Geometry check sheet. Reference: the model listing, model coordinates, mm. Give positions to 0.01 mm unless a question says otherwise; leave off trailing zeros. Write each loop counter-clockwise with the first axis right and the second up, starting at its lowest first coordinate (ties: lowest second). Pieces come first, ordered by that corner, then holes. Notation, with made-up numbers: (47, 57) -> (53, 57) arc R4 cw to (53, 63) -> close; hole circle Ø4 at (46.25, 62.25). An arc over 180 degrees is marked (long way). One line per item, written item: value.
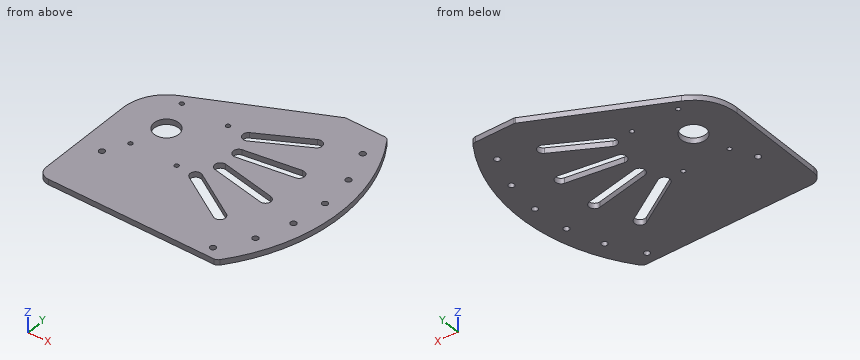
from build123d import *

# Parameters (mm, degrees)
SKETCH1_R           = 3.3782
SKETCH1_R_2         = 14.2875
BOSS_EXTRUDE1_DEPTH = 6.35
FILLET1_R           = 3.175
SKETCH2_R           = 2.54
CUT_EXTRUDE1_DEPTH  = 6.35


with BuildPart() as part:
    # Sketch1 → Boss-Extrude1 (new body)
    with BuildSketch(Plane.XY):
        with BuildLine():
            ThreePointArc((155.542598667, -127), (158.336226208, -126.352468339), (160.56010185, -124.541935484))
            ThreePointArc((160.56010185, -124.541935484), (203.040311847, -8.054301034), (169.920839989, 111.432258065))
            ThreePointArc((169.920839989, 111.432258065), (167.628276357, 113.537255082), (164.61081374, 114.3))
            Line((164.61081374, 114.3), (119.1365603, 114.3))
            Line((119.1365603, 114.3), (-22.183826694, 45.70030452))
            ThreePointArc((-22.183826694, 45.70030452), (-43.055652335, 26.960170659), (-50.8, 0))
            Line((-50.8, 0), (-50.8, -114.3))
            ThreePointArc((-50.8, -114.3), (-47.080256121, -123.280256121), (-38.1, -127))
            Line((-38.1, -127), (155.542598667, -127))
        make_face()
        with Locations((144.383975911, -114.3)):
            Circle(SKETCH1_R, mode=Mode.SUBTRACT)
        with Locations((166.325065928, -79.042592339)):
            Circle(SKETCH1_R, mode=Mode.SUBTRACT)
        with Locations((179.808375328, -39.76541584)):
            Circle(SKETCH1_R, mode=Mode.SUBTRACT)
        with Locations((184.148262492, 1.5342404)):
            Circle(SKETCH1_R, mode=Mode.SUBTRACT)
        with Locations((179.124039222, 42.756241887)):
            Circle(SKETCH1_R, mode=Mode.SUBTRACT)
        with Locations((164.991192987, 81.804402963)):
            Circle(SKETCH1_R, mode=Mode.SUBTRACT)
        with BuildLine():
            Line((63.70579448, 42.288701206), (119.344293443, 72.892743964))
            ThreePointArc((119.344293443, 72.892743964), (127.968547615, 70.389298344), (125.465101994, 61.765044172))
            Line((125.465101994, 61.765044172), (69.826603031, 31.161001414))
            ThreePointArc((69.826603031, 31.161001414), (61.202348859, 33.664447034), (63.70579448, 42.288701206))
        make_face(mode=Mode.SUBTRACT)
        with BuildLine():
            ThreePointArc((61.899520347, -44.891111378), (59.755440765, -36.170565366), (68.475986777, -34.026485785))
            Line((68.475986777, -34.026485785), (122.799114746, -66.908817936))
            ThreePointArc((122.799114746, -66.908817936), (124.943194328, -75.629363948), (116.222648316, -77.77344353))
            Line((116.222648316, -77.77344353), (61.899520347, -44.891111378))
        make_face(mode=Mode.SUBTRACT)
        with BuildLine():
            ThreePointArc((73.520186848, -21.01296328), (68.52280869, -13.551648949), (75.984123021, -8.554270791))
            Line((75.984123021, -8.554270791), (138.277585466, -20.873951654))
            ThreePointArc((138.277585466, -20.873951654), (143.274963624, -28.335265985), (135.813649293, -33.332644143))
            Line((135.813649293, -33.332644143), (73.520186848, -21.01296328))
        make_face(mode=Mode.SUBTRACT)
        with BuildLine():
            ThreePointArc((76.273233773, 5.399658308), (69.025314597, 10.701796332), (74.327452622, 17.949715507))
            Line((74.327452622, 17.949715507), (137.077738619, 27.678621264))
            ThreePointArc((137.077738619, 27.678621264), (144.325657795, 22.37648324), (139.02351977, 15.128564064))
            Line((139.02351977, 15.128564064), (76.273233773, 5.399658308))
        make_face(mode=Mode.SUBTRACT)
        Circle(SKETCH1_R_2, mode=Mode.SUBTRACT)
        with Locations((-25.4, -63.5)):
            Circle(SKETCH1_R, mode=Mode.SUBTRACT)
    extrude(amount=BOSS_EXTRUDE1_DEPTH)

    # Fillet1
    fillet1_edges = [part.edges().sort_by_distance(p)[0] for p in [
        (119.1365603, 114.3, 3.175),
    ]]
    fillet(fillet1_edges, radius=FILLET1_R)

    # Sketch2 → Cut-Extrude1 (cut)
    with BuildSketch(Plane.XY.offset(6.35)):
        with Locations((-12.072682951, 38.1)):
            Circle(SKETCH2_R)
        with Locations((-12.072682951, -38.1)):
            Circle(SKETCH2_R)
        with Locations((41.902317049, -38.1)):
            Circle(SKETCH2_R)
        with Locations((41.902317049, 38.1)):
            Circle(SKETCH2_R)
    extrude(amount=-CUT_EXTRUDE1_DEPTH, mode=Mode.SUBTRACT)


solid = part.part
1) Scan lines: probe 1 along Y at (x, z) = (78, 2.5); probe 2 along Y at (x, z) = (94, 2.5); probe 3 along Y at (x, z) = (137, 4). Record each from-to range of solid material in increasing order.
Verdict:
probe 1: -127 to -54.64, -39.79 to -21.9, -8.95 to 5.67, 18.52 to 35.66, 50.15 to 94.33
probe 2: -127 to -64.32, -49.48 to -25.06, -12.12 to 8.15, 21 to 44.46, 58.95 to 102.1
probe 3: -127 to -33.45, -20.62 to 14.81, 27.67 to 114.3
2) Sectioned sample at C-C on y = -63.5. Record the cut outline in (x, z).
Verdict:
outline: (-50.8, 0) -> (-28.78, 0) -> (-28.78, 6.35) -> (-50.8, 6.35) -> close; (-22.02, 0) -> (92.64, 0) -> (92.64, 6.35) -> (-22.02, 6.35) -> close; (117.17, 0) -> (193.02, 0) -> (193.02, 6.35) -> (117.17, 6.35) -> close
3) Sectioned sample at D-D on x = -25.4. Record the cut outline in (y, z), plus the area to 3 significant figures.
Verdict:
outline: (-127, 0) -> (-66.88, 0) -> (-66.88, 6.35) -> (-127, 6.35) -> close; (-60.12, 0) -> (43.99, 0) -> (43.99, 6.35) -> (-60.12, 6.35) -> close
area: 1,040 mm^2
4) Depth check by flat-ended pin: pin 1 Ø1.5 at (y, z) = (56, 4) entering from -X; pin 2 Ø1.5 at (y, z) = (-50, 3) entering from +X. Enter the tip coordinate at first touch or a pass-through.
Verdict:
pin 1: x = -2.51
pin 2: x = 197.14
5) Sectioned sample at A-A on x = 91.5. Record the cut outline in (y, z).
Verdict:
outline: (-127, 0) -> (-62.81, 0) -> (-62.81, 6.35) -> (-127, 6.35) -> close; (-47.96, 0) -> (-24.57, 0) -> (-24.57, 6.35) -> (-47.96, 6.35) -> close; (-11.62, 0) -> (7.76, 0) -> (7.76, 6.35) -> (-11.62, 6.35) -> close; (20.61, 0) -> (43.08, 0) -> (43.08, 6.35) -> (20.61, 6.35) -> close; (57.58, 0) -> (100.88, 0) -> (100.88, 6.35) -> (57.58, 6.35) -> close
6) Sectioned sample at B-B on x = 5.5. Record the cut outline in (y, z).
Verdict:
outline: (-127, 0) -> (-13.19, 0) -> (-13.19, 6.35) -> (-127, 6.35) -> close; (13.19, 0) -> (59.14, 0) -> (59.14, 6.35) -> (13.19, 6.35) -> close
